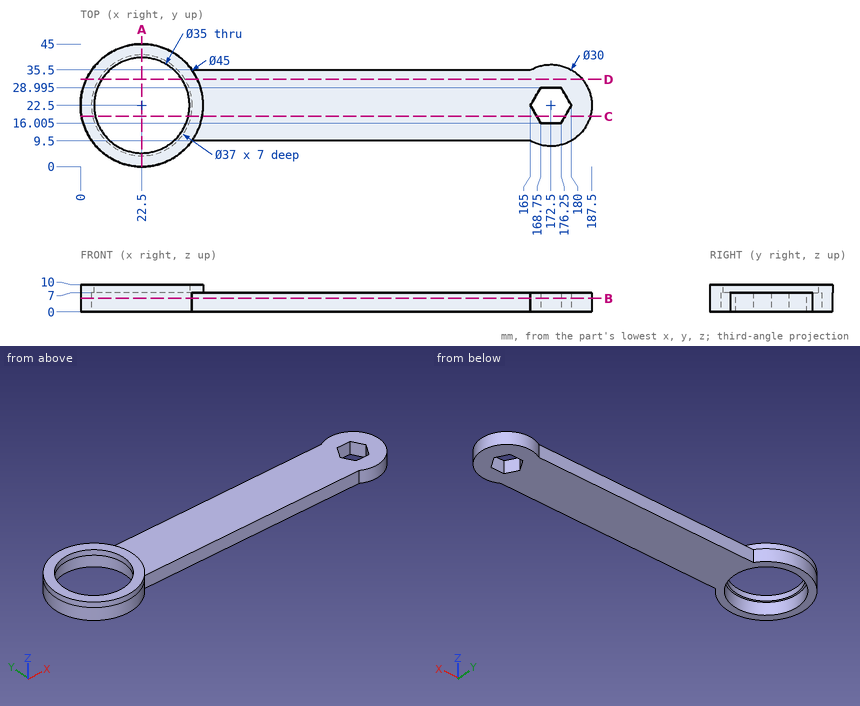
Source: three-view drawing plus pictorial views. Frame: mm from the lowest corner of the part. Coordinates: 2 decimals unless noted, no trailing zeros. Order: outer loops, then holes, each group sorted by start corner. A loop starts at its lowest first (then second) coordinate and runs counter-clockwise, first axis right, second up.
1) Section B-B (z = 5). Give the number of separate pieces and of enclosed holes in the cut face, then the cut area to 3 significant figures.
Result sheet:
separate pieces: 1
enclosed holes: 2
area: 4,090 mm2
2) Section D-D (y = 32). Return loops of the section in (x, z).
Result sheet:
outline: (2.1, 0) - (6.63, 0) - (6.63, 7) - (7.8, 7) - (7.8, 10) - (2.1, 10) - close; (37.2, 7) - (38.37, 7) - (38.37, 0) - (184.11, 0) - (184.11, 7) - (42.9, 7) - (42.9, 10) - (37.2, 10) - close
3) First-contact query: P1, Ø8, axis at x = 160.5, y = 22.5, coming from the +Z side; P2, Ø6, axis at x = 55, z = 6, coming from the -Y side; P3, Ø5.5, axis at x = 171, z = 4.5, coming from the +Y side; P4, Ø4, axis at x = 21, z = 7.5, coming from the +Y side. Flat tips, straight axial feed; report the tip coordinate or a pass-through.
Result sheet:
P1: stops at z = 7
P2: stops at y = 9.5
P3: stops at y = 37.5
P4: stops at y = 45
4) Section A-A (x = 22.5). Return loops of the section in (y, z), then the cut area to 3 significant figures.
Result sheet:
outline: (0, 0) - (4, 0) - (4, 7) - (5, 7) - (5, 10) - (0, 10) - close; (40, 7) - (41, 7) - (41, 0) - (45, 0) - (45, 10) - (40, 10) - close
area: 86.0 mm2
5) Ray query, probe 1 along Y at (x, z) = (22.5, 9.2); probe 2 along Y at (x, z) = (22.5, 4.75); probe 3 along X at (y, z) = (36, 4). Return the intervals inside material, ascending.
Result sheet:
probe 1: y = 0 to 5, 40 to 45
probe 2: y = 0 to 4, 41 to 45
probe 3: x = 4.5 to 9.85, 35.15 to 40.5, 165.96 to 179.04
6) Section C-C (y = 18.5). Return loops of the section in (x, z), then the cut area to 3 significant figures.
Result sheet:
outline: (0.36, 0) - (4.44, 0) - (4.44, 7) - (5.46, 7) - (5.46, 10) - (0.36, 10) - close; (39.54, 7) - (40.56, 7) - (40.56, 0) - (167.31, 0) - (167.31, 7) - (44.64, 7) - (44.64, 10) - (39.54, 10) - close; (177.69, 0) - (186.96, 0) - (186.96, 7) - (177.69, 7) - close
area: 1,010 mm2
